The listing builds one solid part. Answer for the finished solid, in the listing's coordinates (mm). Round coordinates to 2 decimals unless told otherwise and drop trailing zeros. Loops run counter-clockwise (first coordinate to the right, second up) from the corner with the lowest first, then second, coordinate; pieces in that order, holes last. Notation, with made-up numbers: (10.5, 24.5) -> (25.5, 24.5) arc R26 ccw to (25.5, 59.5) -> close; hole circle Ø7 at (-20, 76.25). An arc over 180 degrees is marked (long way). One line per question, with ' | ' between items.
from build123d import *


with BuildPart() as part:
    # Esboço1 → Revolução1 (revolve)
    with BuildSketch(Plane.XY, mode=Mode.PRIVATE) as revolu_o1_sk:
        with BuildLine():
            Line((-1.025, 5.08), (-0.51, 0))
            Line((-0.51, 0), (0, 0))
            Line((0, 0), (0, 31.5))
            ThreePointArc((0, 31.5), (-0.237708503, 31.439880288), (-0.418253138, 31.273978671))
            ThreePointArc((-0.418253138, 31.273978671), (-0.987090573, 30.091270748), (-1.228582631, 28.801287941))
            ThreePointArc((-1.228582631, 28.801287941), (-1.244644702, 28.400787059), (-1.25, 28))
            Line((-1.25, 28), (-1.25, 26.8))
            ThreePointArc((-1.25, 26.8), (-1.084829578, 26.619588497), (-1.025, 26.382417673))
            Line((-1.025, 26.382417673), (-1.025, 5.08))
        make_face()
    revolve(revolu_o1_sk.sketch.rotate(Axis((0, 0, 0), (0, 1, 0)), 270), axis=Axis((0, 0, 0), (0, 1, 0)))


solid = part.part
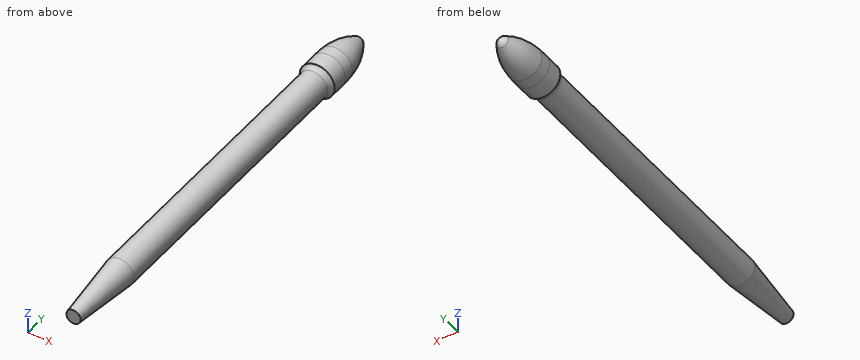
Q1. Given pin 1 Ø1.5 at (x, y) = (-0.5, 5) entering from +Z (3 decimals); pin 2 Ø1 at (y, z) = (11, 0.5) entering from +X (3 decimals), each flat-ended and moving along its own axis, determine where each tip first touches the part or whether it passes through.
Numbers:
pin 1: z = 1.025 | pin 2: x = 1.025
Q2. Find the intervals of material crossed by line 1 (Z direction, x = 0.1, y = 8.5); line 2 (Z direction, x = -0.5, y = 16), in increasing order. Write a range as from..to.
Numbers:
line 1: -1.02..1.02 | line 2: -0.89..0.89
Q3. A cutting plane is placed at A-A on y = 7.5. Give the vertices of the cut face in (x, z) (3 decimals).
Numbers:
outline: circle Ø2.05 at (0, 0)
